```python
from build123d import *

# Parameters (mm, degrees)
F0_W     = 63.5
F0_H     = 63.5
F1_DEPTH = 3.175
F2_W     = 63.5
F2_H     = 3.175
F3_DEPTH = 50.8
F5_DEPTH = 63.5


with BuildPart() as f1:
    # F0 (on Top) → F1 (new body)
    with BuildSketch(Plane.XY):
        with Locations((-31.75, -31.75)):
            Rectangle(F0_W, F0_H)
    extrude(amount=F1_DEPTH)

    # F2 (on face) → F3 (join)
    with BuildSketch(Plane.XY.offset(3.175)):
        with Locations((-31.75, -61.9125)):
            Rectangle(F2_W, F2_H)
    extrude(amount=F3_DEPTH)

    # F4 (on face) → F5 (cut)
    with BuildSketch(Plane(origin=(-63.5, 0, 0), x_dir=(0, -1, 0), z_dir=(-1, 0, 0))):
        Polygon((61.9125, 53.975), (63.5, 3.175), (63.5, 53.975), align=None)
    extrude(amount=-F5_DEPTH, mode=Mode.SUBTRACT)


solid = f1.part
```
The model under review builds one solid part; all positions refer to its coordinate system, in mm. A direction names the side the tool comes from. Give positions to 0.01 mm unless a question says otherwise; leave off trailing zeros. Write each loop counter-clockwise with the first axis right and the second up, starting at its lowest first coordinate (ties: lowest second). Pieces come first, ordered by that corner, then holes. Notation, with made-up numbers: (67, -4.5) -> (106, -4.5) arc R11 cw to (106, 5.5) -> close; hole circle Ø2 at (20, 84). An arc over 180 degrees is marked (long way). Answer in a Markdown table with one row per item.
1) Add section B-B on y = -54.5. State the section outline as (x, z) points (3 decimals), plus the area to 3 significant figures.
Worked answers:
| item | result |
|---|---|
| outline | (-63.5, 0) -> (0, 0) -> (0, 3.175) -> (-63.5, 3.175) -> close |
| area | 202 mm² |
2) Add section A-A on x = -36. State the section outline as (y, z) points (1 decimal).
Worked answers:
| item | result |
|---|---|
| outline | (-63.5, 0) -> (0, 0) -> (0, 3.2) -> (-60.3, 3.2) -> (-60.3, 54) -> (-61.9, 54) -> (-63.5, 3.2) -> close |
3) Tool access review of faces 1 (the flat face through (-32, 0, 2)), 2 (the flat face through (-32, -30, 3.175)): name each direction out of +Z, -Z, +X, -X, +Y, -Y from which nothing blocks a thin tool from reaching the whole face with its end or side.
Worked answers:
| item | result |
|---|---|
| face 1 | +Z, -Z, +X, -X, +Y |
| face 2 | +Z, +X, -X, +Y |
4) Add section C-C on z = 38. State the section outline as (x, y) points (3 decimals).
Worked answers:
| item | result |
|---|---|
| outline | (-63.5, -62.412) -> (0, -62.412) -> (0, -60.325) -> (-63.5, -60.325) -> close |
5) For L1, parallel to Z at x = -43.5, y = -4.5 (3 decimals); L2, parallel to Y at x = -58, z = 50 (3 decimals); L3, parallel to Y at x = -44.5, z = 23 (3 decimals), list the stretches that pass through material, from the lowest coordinate up. Write a range as [from, to].
Worked answers:
| item | result |
|---|---|
| L1 | [0, 3.175] |
| L2 | [-62.037, -60.325] |
| L3 | [-62.88, -60.325] |
6) Clearance check with flat-ended pins moving along their axes: P1, Ø3, axis at x = -13.5, y = -13.5, coming from the +Z side (3 decimals); P2, Ø4, axis at x = -30.5, z = 28, coming from the +Y side (3 decimals); P3, Ø8, axis at x = -35.5, y = -35.5, coming from the -Z side; P4, Ø10, axis at y = -23.5, z = 13, coming from the +X side. State where each tip first meets the part, or that it passes through.
Worked answers:
| item | result |
|---|---|
| P1 | z = 3.175 |
| P2 | y = -60.325 |
| P3 | z = 0 |
| P4 | through |
